Geometry: final body of the model. Coordinates: model frame, mm. A direction names the side the tool comes from. Give positions to 0.01 mm unless a question says otherwise; leave off trailing zeros. Write each loop counter-clockwise with the first axis right and the second up, starting at its lowest first coordinate (ties: lowest second). Pieces come first, ordered by that corner, then holes. Notation, with made-up numbers: (16, 57.25) -> (24, 57.25) arc R16 cw to (24, 74.25) -> close; hole circle Ø4 at (51.25, -33). An arc over 180 degrees is marked (long way). Answer in a Markdown table with one row per item. Add a question column.
from build123d import *

# Parameters (mm, degrees)
SZKIC1_R                    = 27.5
SZKIC1_W                    = 48
SZKIC1_H                    = 30
DODANIE_WYCI_GNI_CIE1_DEPTH = 3
SZKIC2_R                    = 27.5
DODANIE_WYCI_GNI_CIE2_DEPTH = 55
SZKIC3_R                    = 26
WYTNIJ_WYCI_GNI_CIE1_DEPTH  = 10
SZKIC4_R                    = 21
DODANIE_WYCI_GNI_CIE3_DEPTH = 10
DODANIE_WYCI_GNI_CIE3_TAPER = -15
WYTNIJ_WYCI_GNI_CIE2_REACH  = 5
SZKIC5_R                    = 2.25
ZAOKR_GLENIE1_R             = 4


with BuildPart() as part:
    # Szkic1 → Dodanie-wyciągnięcie1 (new body)
    with BuildSketch(Plane.XY):
        Circle(SZKIC1_R)
        with Locations((0, 28.425721582)):
            Rectangle(SZKIC1_W, SZKIC1_H)
    extrude(amount=DODANIE_WYCI_GNI_CIE1_DEPTH)

    # Szkic2 → Dodanie-wyciągnięcie2 (add)
    with BuildSketch(Plane.XY.offset(3)):
        Circle(SZKIC2_R)
    extrude(amount=DODANIE_WYCI_GNI_CIE2_DEPTH)

    # Szkic3 → Wytnij-wyciągnięcie1 (cut)
    with BuildSketch(Plane.XY.offset(58)):
        Circle(SZKIC3_R)
    extrude(amount=-WYTNIJ_WYCI_GNI_CIE1_DEPTH, mode=Mode.SUBTRACT)

    # Szkic4 → Dodanie-wyciągnięcie3 (add)
    with BuildSketch(Plane.XY.offset(48)):
        Circle(SZKIC4_R)
    extrude(amount=DODANIE_WYCI_GNI_CIE3_DEPTH, taper=DODANIE_WYCI_GNI_CIE3_TAPER)

    # Szkic5 → Wytnij-wyciągnięcie2 (cut, up to next)
    with BuildSketch(Plane.XY.offset(3), mode=Mode.PRIVATE) as wytnij_wyci_gni_cie2_sk1:
        with Locations((-20, 39.425721582)):
            Circle(SZKIC5_R)
    wytnij_wyci_gni_cie2_tool1 = extrude(wytnij_wyci_gni_cie2_sk1.sketch, amount=-WYTNIJ_WYCI_GNI_CIE2_REACH, mode=Mode.PRIVATE) & part.part
    add(wytnij_wyci_gni_cie2_tool1.solids().sort_by_distance((-20, 39.425722, 3))[0], mode=Mode.SUBTRACT)
    # Szkic5 → Wytnij-wyciągnięcie2 (cut, up to next)
    with BuildSketch(Plane.XY.offset(3), mode=Mode.PRIVATE) as wytnij_wyci_gni_cie2_sk2:
        with Locations((20, 39.425721582)):
            Circle(SZKIC5_R)
    wytnij_wyci_gni_cie2_tool2 = extrude(wytnij_wyci_gni_cie2_sk2.sketch, amount=-WYTNIJ_WYCI_GNI_CIE2_REACH, mode=Mode.PRIVATE) & part.part
    add(wytnij_wyci_gni_cie2_tool2.solids().sort_by_distance((20, 39.425722, 3))[0], mode=Mode.SUBTRACT)

    # Zaokrąglenie1
    zaokr_glenie1_edges = [part.edges().sort_by_distance(p)[0] for p in [
        (24, 43.425721582, 1.5),
        (-24, 43.425721582, 1.5),
    ]]
    fillet(zaokr_glenie1_edges, radius=ZAOKR_GLENIE1_R)


solid = part.part
Q1. Section A-A on z = 10.5. Return loops of the section in (x, y).
Q2. Line query: probe 1 along X at (y, z) = (-16, 52); probe 2 along X at (y, z) = (-12, 49); probe 3 along Z at (x, y) = (4.5, 24.5). Output: solid intervals per line, ascending. Write a range as from..to.
Q3. Access query for faces 5 (the flat face through (-24, 26, 1)), 6 (the cylindrical face through (-20.633, -15.821, 53.07)), 7 (the flat face through (24, 26, 1)), 8 (the conical face through (-4.589, -20.664, 48.626)), 9 (the flat face through (0, 0, 58)). Directions: +Z, -Z, +X, -X, +Y, -Y. A direction counts if a zero-diameter tool reaches every point of the face in a straight line with its end or side. Return the directions, or none.
Q4. Pull-direction query (Z, two-part tool) for faces 1 (the flat face through (0, 8, 0)), 2 (the flat face through (1.8, 21.3, 48)), 3 (the cylindrical face through (-17.854, 40.102, 1.521)), 4 (the flat face through (10.1, -24.3, 58)); classes: +Z half, -Z half, draft (parallel to the pull), parting line (faces both ways), or undercut.
Q5. Contact query for flat-ended pins moving along their axis: pin 1 Ø10 at (x, z) = (20.5, 29.5) entering from +Y; pin 2 Ø5 at (x, z) = (-2, 18.5) entering from -Y; pin 3 Ø3 at (y, z) = (9, 6) entering from +X. Output: stop coordinate, or through.
Checks:
| question | item | result |
|---|---|---|
| 1 | outline | circle Ø55 at (0, 0) |
| 2 | probe 1 | -22.37..-20.49, -15.2..15.2, 20.49..22.37 |
| 2 | probe 2 | -24.74..-23.07, -17.56..17.56, 23.07..24.74 |
| 2 | probe 3 | 0..48 |
| 3 | face 5 | +Z, -Z, -X, +Y |
| 3 | face 6 | +Z |
| 3 | face 7 | +Z, -Z, +X, +Y |
| 3 | face 8 | none |
| 3 | face 9 | +Z, +X, -X, +Y, -Y |
| 4 | face 1 | -Z half |
| 4 | face 2 | undercut |
| 4 | face 3 | draft |
| 4 | face 4 | +Z half |
| 5 | pin 1 | y = 22.72 |
| 5 | pin 2 | y = -27.5 |
| 5 | pin 3 | x = 26.46 |
